Check sheet for the modelled part. Datum: model origin and axes. Units: mm. Face numbers are marked on the shaded views. A direction names the side the tool comes from. Give positions to 0.01 mm unless a question says otherwise; leave off trailing zeros. Write each loop counter-clockwise with the first axis right and the second up, starting at its lowest first coordinate (ties: lowest second). Pieces come first, ordered by that corner, then holes.
from build123d import *

# Parameters (mm, degrees)
SKETCH_1_R               = 11
EXTRUDE_2_DEPTH          = 3.5
SKETCH_2_R               = 5.15
EXTRUDE_3_DEPTH          = 11
CUT_EXTRUDE_1_DEPTH      = 22.266170318
CUT_EXTRUDE_1_DEPTH_BACK = 22.266170318
SKETCH_3_R               = 4
CUT_EXTRUDE_4_REACH      = 23.266
SKETCH_4_R               = 1.75
PATTERN_CIRCULAR_6_COUNT = 4
SKETCH_7_R               = 5
EXTRUDE_4_DEPTH          = 1.5
SKETCH_8_R               = 3.535076685
CUT_EXTRUDE_5_DEPTH      = 23.315913604


with BuildPart() as part:
    # 草图1 → 凸台-拉伸2 (new body)
    with BuildSketch(Plane(origin=(0, 0, 0), x_dir=(1, 0, 0), z_dir=(0, 1, 0))):
        with Locations(Location((0, 0, 0), (0, 0, 270))):
            Circle(SKETCH_1_R)
    extrude(amount=EXTRUDE_2_DEPTH)

    # 草图2 → 凸台-拉伸3 (add)
    with BuildSketch(Plane.XZ):
        with Locations(Location((0, 0, 0), (0, 0, 90))):
            Circle(SKETCH_2_R)
    extrude(amount=EXTRUDE_3_DEPTH)

    # 草图3 → 切除-拉伸1 (cut, two sides: drawn at the far end of the back side and taken through both)
    with BuildSketch(Plane.XZ.offset(11).offset(-CUT_EXTRUDE_1_DEPTH_BACK)):
        with Locations(Location((0, 0, 0), (0, 0, 270))):
            Circle(SKETCH_3_R)
    extrude(amount=CUT_EXTRUDE_1_DEPTH + CUT_EXTRUDE_1_DEPTH_BACK, mode=Mode.SUBTRACT)

    # 草图4 → 切除-拉伸4 (cut, up to next)
    with BuildSketch(Plane(origin=(0, 3.5, 0), x_dir=(1, 0, 0), z_dir=(0, 1, 0)), mode=Mode.PRIVATE) as cut_extrude_4_sk1:
        with Locations(Location((0, 8, 0), (0, 0, 270))):
            Circle(SKETCH_4_R)
    cut_extrude_4_tool1 = extrude(cut_extrude_4_sk1.sketch, amount=-CUT_EXTRUDE_4_REACH, mode=Mode.PRIVATE) & part.part
    cut_extrude_4 = cut_extrude_4_tool1.solids().sort_by_distance((0, 3.5, -8))[0]
    add(cut_extrude_4, mode=Mode.SUBTRACT)

    # 阵列(圆周)6: 切除-拉伸4 ×4 about axis
    pattern_circular_6_axis = Axis((0, 0, 0), (0, 1, 0))
    for i in range(1, PATTERN_CIRCULAR_6_COUNT):
        add(cut_extrude_4.rotate(pattern_circular_6_axis, i * 360 / PATTERN_CIRCULAR_6_COUNT), mode=Mode.SUBTRACT)

    # 草图7 → 凸台-拉伸4 (add)
    with BuildSketch(Plane(origin=(0, 3.5, 0), x_dir=(1, 0, 0), z_dir=(0, 1, 0))):
        with Locations(Location((0, 0, 0), (0, 0, 270))):
            Circle(SKETCH_7_R)
    extrude(amount=EXTRUDE_4_DEPTH)

    # 草图8 → 切除-拉伸5 (cut, through all)
    with BuildSketch(Plane(origin=(0, 5, 0), x_dir=(1, 0, 0), z_dir=(0, 1, 0))):
        with Locations(Location((0, 0, 0), (0, 0, 270))):
            Circle(SKETCH_8_R)
    extrude(amount=-CUT_EXTRUDE_5_DEPTH, mode=Mode.SUBTRACT)


solid = part.part
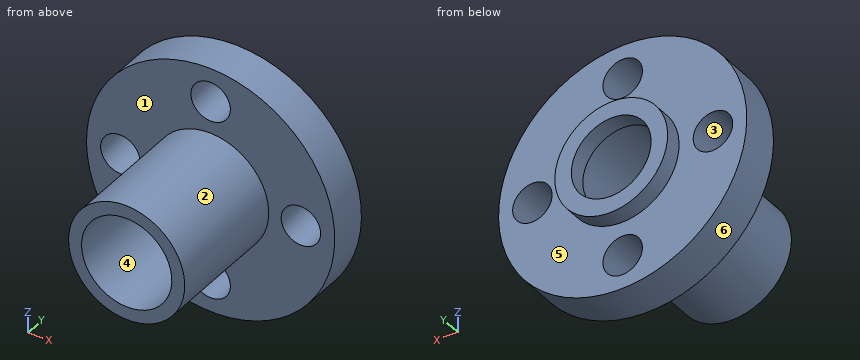
1) Scan lines: L1, parallel to X at y = -5.25, z = 0; L2, parallel to X at y = 3.85, z = 0; L3, parallel to Z at x = -3.5, y = -0.5. Record each from-to range of solid material in increasing order.
2) Sectioned sample at C-C on y = 0.5. Record the boundary of the cut face in (x, z), then the cut area to 3 significant figures.
3) Sectioned sample at D-D on x = -7.5. Record the boundary of the cut face in (y, z), then the cut area to 3 significant figures.
4) Sectioned sample at B-B on x = 0. Record the boundary of the cut face in (y, z).
5) Gauge pin test, flat ends, axial feed: pin 1 (1.5 mm diameter, centred on y = -7, z = 5.5, fed in from -X); pin 2 (2 mm diameter, centred on x = 0, z = -8, fed in from +Y); pin 3 (6 mm diameter, centred on x = 0.5, y = -9.5, fed in from -Z); pin 4 (8 mm diameter, centred on y = -3, z = -5.5, fed in from +X). Record the tip position at first contact, or that the pin passes through.
6) Access from +Z, -Z, +X, -X, +Y, -Y to the whole of each face (thin tool, end or side, straight path). Record for the marked faces 4, 5 and 6.
7) Sectioned sample at A-A on z = 0. Record the boundary of the cut face in (x, y).
8) Draft check along X on the marked faces 1, 2 and 3. Enter one of: +X half, -X half, draft (parallel to the pull), parting line (faces both ways), or undercut.
Answers below:
1. L1: x = -5.15 to -4, 4 to 5.15
1. L2: x = -5 to -3.54, 3.54 to 5
1. L3: z = -3.78 to -1.94, 1.94 to 3.78
2. outline: circle Ø22 at (0, 0); hole circle Ø3.5 at (-8, 0); hole circle Ø8 at (0, 0); hole circle Ø3.5 at (0, -8); hole circle Ø3.5 at (0, 8); hole circle Ø3.5 at (8, 0)
2. area: 291 mm2
3. outline: (0, -8.05) - (3.5, -8.05) - (3.5, -1.68) - (0, -1.68) - close; (0, 1.68) - (3.5, 1.68) - (3.5, 8.05) - (0, 8.05) - close
3. area: 44.6 mm2
4. outline: (-11, -5.15) - (0, -5.15) - (0, -6.25) - (3.5, -6.25) - (3.5, -5) - (5, -5) - (5, -3.54) - (3.5, -3.54) - (3.5, -4) - (-11, -4) - close; (-11, 4) - (3.5, 4) - (3.5, 3.54) - (5, 3.54) - (5, 5) - (3.5, 5) - (3.5, 6.25) - (0, 6.25) - (0, 5.15) - (-11, 5.15) - close; (0, -11) - (3.5, -11) - (3.5, -9.75) - (0, -9.75) - close; (0, 9.75) - (3.5, 9.75) - (3.5, 11) - (0, 11) - close
5. pin 1: stops at x = -1.99
5. pin 2: passes through
5. pin 3: stops at z = -5.15
5. pin 4: stops at x = 10.62
6. face 4: -Y
6. face 5: +Y
6. face 6: +Y, -Y
7. outline: (-11, 0) - (-9.75, 0) - (-9.75, 3.5) - (-11, 3.5) - close; (-6.25, 0) - (-5.15, 0) - (-5.15, -11) - (-4, -11) - (-4, 3.5) - (-3.54, 3.5) - (-3.54, 5) - (-5, 5) - (-5, 3.5) - (-6.25, 3.5) - close; (3.54, 3.5) - (4, 3.5) - (4, -11) - (5.15, -11) - (5.15, 0) - (6.25, 0) - (6.25, 3.5) - (5, 3.5) - (5, 5) - (3.54, 5) - close; (9.75, 0) - (11, 0) - (11, 3.5) - (9.75, 3.5) - close
8. face 1: draft
8. face 2: parting line
8. face 3: undercut
